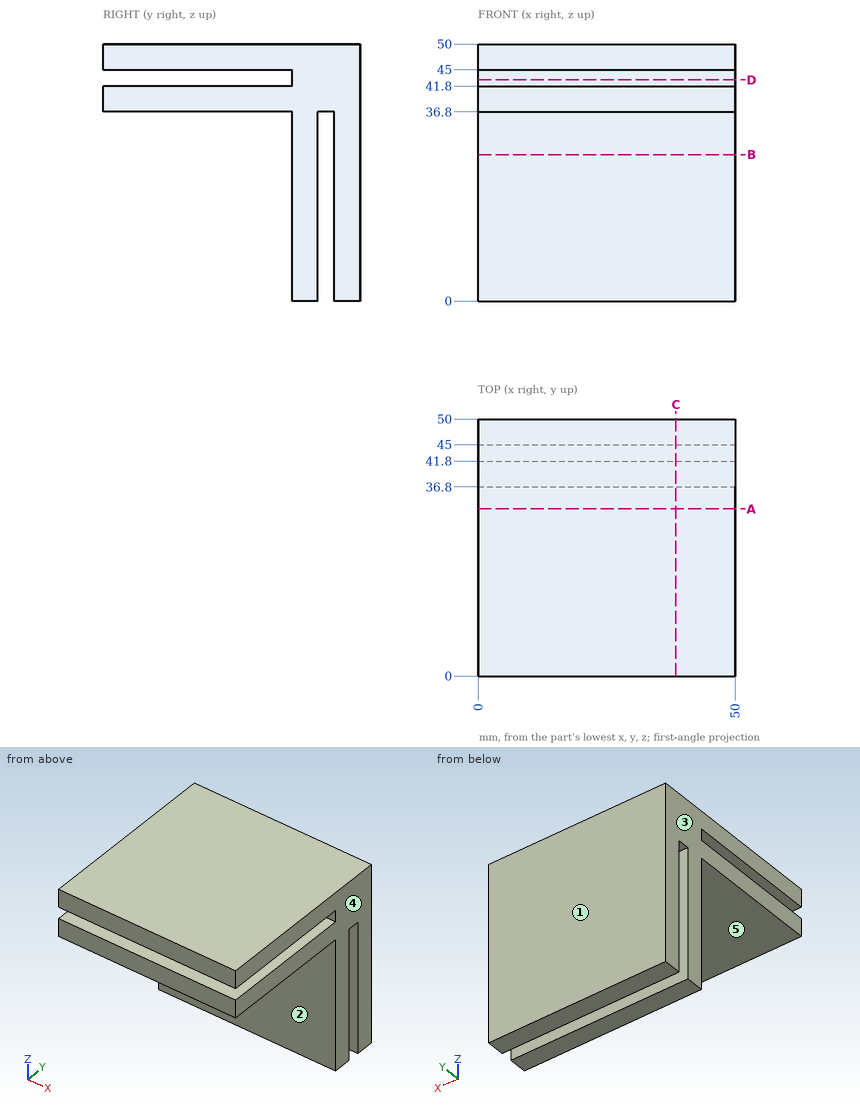
Input: dimensioned drawing with shaded views. Units: mm. Origin: part minimum x, y, z. A direction names the side the tool comes from. Coordinates: 2 decimals unless noted, no trailing zeros. Loops run counter-clockwise (first coordinate to the right, second up) from the corner with the lowest first, then second, coordinate; pieces in that order, holes last. Notation, with made-up numbers: (-14.5, 38) -> (0.5, 38) arc R25 ccw to (0.5, 71) -> close; hole circle Ø6 at (-26, 87). An arc over 180 degrees is marked (long way). Use a Markdown table: item, result. Add a question column.
(1) Line query: line 1 along Y through (x, z) = (11.5, 17.5); line 2 along Z through (x, y) = (2.5, 43). Output: solid intervals per line, ascending.
(2) Section query D-D, the plane z = 43. Return loops of the section in (x, y).
(3) Access query for the marked faces 1 and 2. Directions: +Z, -Z, +X, -X, +Y, -Y. A direction counts if a zero-diameter tool reaches every point of the face in a straight line with its end or side. Return the directions, or none.
(4) Pin query (flat end, axial travel): pin 1 Ø1 at (x, z) = (15, 43) entering from -Y; pin 2 Ø1.6 at (x, y) = (23, 43.5) entering from -Z. Return the tip coordinate at first contact, or that it passes through.
(5) Mould query, pull axis X, two halves, no side actions, for the marked faces 3, 4 and 5. Classes: pulls with the +X half, pulls with the -X half, needs draft (parallel to the pull), parting line crosses it, or undercut.
(6) Section query C-C, the plane x = 38.5. Return loops of the section in (y, z), plus the area to 3 significant figures.
(7) Section query A-A, the plane y = 32.5. Return loops of the section in (x, z), plus the area to 3 significant figures.
Answer:
| question | item | result |
|---|---|---|
| 1 | line 1 | y = 36.8 to 41.8, 45 to 50 |
| 1 | line 2 | z = 36.8 to 50 |
| 2 | outline | (0, 36.8) -> (50, 36.8) -> (50, 50) -> (0, 50) -> close |
| 3 | face 1 | +Z, -Z, +X, -X, +Y |
| 3 | face 2 | -Z, +X, -X, -Y |
| 4 | pin 1 | stops at y = 36.8 |
| 4 | pin 2 | stops at z = 36.8 |
| 5 | face 3 | pulls with the -X half |
| 5 | face 4 | pulls with the +X half |
| 5 | face 5 | needs draft |
| 6 | outline | (0, 36.8) -> (36.8, 36.8) -> (36.8, 0) -> (41.8, 0) -> (41.8, 36.8) -> (45, 36.8) -> (45, 0) -> (50, 0) -> (50, 50) -> (0, 50) -> (0, 45) -> (36.8, 45) -> (36.8, 41.8) -> (0, 41.8) -> close |
| 6 | area | 910 mm^2 |
| 7 | outline | (0, 36.8) -> (50, 36.8) -> (50, 41.8) -> (0, 41.8) -> close; (0, 45) -> (50, 45) -> (50, 50) -> (0, 50) -> close |
| 7 | area | 500 mm^2 |
